Design review of the part built by this model. Coordinates are the model's own, in mm. Face numbers are marked on the shaded views. A direction names the side the tool comes from. Give positions to 0.01 mm unless a question says otherwise; leave off trailing zeros. Loops run counter-clockwise (first coordinate to the right, second up) from the corner with the lowest first, then second, coordinate; pieces in that order, holes last. Notation, with made-up numbers: M 40.25,30 L 79.25,30 A25 ccw 79.25,55 Z; hole C 19,19.5 d7. An arc over 180 degrees is marked long. Answer as CSV lines item,"result".
Autodesk Inventor part; units mm, degrees
ref_plane "YZ Plane" through (0, 0, 0) normal (1, 0, 0) x (0, 1, 0)
ref_plane "XZ Plane" through (0, 0, 0) normal (0, 1, 0) x (-1, 0, 0)
ref_plane "XY Plane" through (0, 0, 0) normal (0, 0, 1) x (1, 0, 0)
sketch "Sketch1" plane through (0, 0, 0) normal (0, 1, 0) x (-1, 0, 0)
  line L0 (0, 0) -> (56, 0)
  line L1 (56, -6.2) -> (56, -90.8)
  line L2 (56, -97) -> (0, -97)
  line L3 (0, -90.8) -> (0, -6.2)
  line L4 (0, 0) -> (-3.5, 0)
  line L5 (-4.5, -1) -> (-4.5, -4.2)
  line L6 (-3.5, -5.2) -> (-1, -5.2)
  line L7 (28, 0) -> (28, -97)
  circle A0 centre (-2.5, -2.6) radius 1.5
  arc A1 (-3.5, 0) -> (-4.5, -1) centre (-3.5, -1) ccw
  arc A2 (-4.5, -4.2) -> (-3.5, -5.2) centre (-3.5, -4.2) ccw
  arc A3 (0, -6.2) -> (-1, -5.2) centre (-1, -6.2) ccw
  line L8 (56, 0) -> (59.5, 0)
  line L9 (60.5, -1) -> (60.5, -4.2)
  line L10 (59.5, -5.2) -> (57, -5.2)
  circle A4 centre (58.5, -2.6) radius 1.5
  arc A5 (60.5, -1) -> (59.5, 0) centre (59.5, -1) ccw
  arc A6 (59.5, -5.2) -> (60.5, -4.2) centre (59.5, -4.2) ccw
  arc A7 (57, -5.2) -> (56, -6.2) centre (57, -6.2) ccw
  line L11 (56, -48.5) -> (0, -48.5)
  line L12 (0, -97) -> (-3.5, -97)
  line L13 (-4.5, -96) -> (-4.5, -92.8)
  line L14 (-3.5, -91.8) -> (-1, -91.8)
  circle A8 centre (-2.5, -94.4) radius 1.5
  arc A9 (-4.5, -96) -> (-3.5, -97) centre (-3.5, -96) ccw
  arc A10 (-3.5, -91.8) -> (-4.5, -92.8) centre (-3.5, -92.8) ccw
  arc A11 (-1, -91.8) -> (0, -90.8) centre (-1, -90.8) ccw
  arc A12 (56, -90.8) -> (57, -91.8) centre (57, -90.8) ccw
  line L15 (59.5, -91.8) -> (57, -91.8)
  line L16 (56, -97) -> (59.5, -97)
  circle A13 centre (58.5, -94.4) radius 1.5
  arc A14 (60.5, -92.8) -> (59.5, -91.8) centre (59.5, -92.8) ccw
  line L17 (60.5, -96) -> (60.5, -92.8)
  arc A15 (59.5, -97) -> (60.5, -96) centre (59.5, -96) ccw
  point P0 (-4.5, 0)
  point P1 (-4.5, -5.2)
  point P2 (0, -5.2)
  point P3 (60.5, 0)
  point P4 (60.5, -5.2)
  point P5 (56, -5.2)
  point P6 (-4.5, -97)
  point P7 (-4.5, -91.8)
  point P8 (0, -91.8)
  point P9 (56, -91.8)
  point P10 (60.5, -91.8)
  point P11 (60.5, -97)
  dimension "d0" = 56
  dimension "d1" = 97
  dimension "d2" = 4.5
  dimension "d3" = 5.2
  dimension "d10" = 1
  dimension "d11" = 1
  dimension "d12" = 2
  dimension "d13" = 2.6
  dimension "d14" = 3
  dimension "d15" = 56
extrude "Vetronite" add sketch "Sketch1" along normal blind 1.7
sketch "Sketch2" plane through (0, 1.7, 0) normal (0, 1, 0) x (1, 0, 0)
  line L0 (-59.5, 0) -> (3.5, 0)
  line L1 (-28, 0) -> (-28, 97)
  line L2 (3.5, 97) -> (-59.5, 97)
  line L3 (-56, 90.8) -> (-56, 6.2)
  line L4 (-56, 48.5) -> (0, 48.5)
  line L5 (0, 6.2) -> (0, 90.8)
  line L6 (-56, 6) -> (0, 6)
  line L7 (0, 6) -> (0, 91)
  line L8 (0, 91) -> (-56, 91)
  line L9 (-56, 91) -> (-56, 6)
  point P0 (0, 0)
  point P1 (-56, 6.2)
  dimension "d16" = 85
  dimension "d17" = 56
extrude "Display" add sketch "Sketch2" along normal blind 3.6
sketch "Sketch3" plane through (0, 0, 0) normal (0, -1, 0) x (1, 0, 0)
  line L0 (-53.3, -4) -> (-2.7, -4)
  line L1 (-2.7, -4) -> (-2.7, -1.5)
  line L2 (-2.7, -1.5) -> (-53.3, -1.5)
  line L3 (-53.3, -1.5) -> (-53.3, -4)
  line L4 (-59.5, 0) -> (3.5, 0)
  line L5 (3.5, -97) -> (-59.5, -97)
  line L6 (-28, -97) -> (-28, 0)
  line L7 (-59.5, 0) -> (3.5, 0)
  point P0 (0, 0)
  dimension "d20" = 50.6
  dimension "d21" = 2.5
  dimension "d22" = 1.5
extrude "Pin" add sketch "Sketch3" along normal blind 8.5
sketch "Sketch4" plane through (0, 0, 0) normal (0, -1, 0) x (1, 0, 0)
  line L0 (-5, -82) -> (-21, -82)
  line L1 (-21, -82) -> (-21, -68)
  line L2 (-21, -68) -> (-5, -68)
  line L3 (-5, -68) -> (-5, -82)
  line L4 (-50, -69) -> (-38, -69)
  line L5 (-38, -69) -> (-38, -57)
  line L6 (-38, -57) -> (-50, -57)
  line L7 (-50, -57) -> (-50, -69)
  line L8 (-36, -69) -> (-24, -69)
  line L9 (-24, -69) -> (-24, -57)
  line L10 (-24, -57) -> (-36, -57)
  line L11 (-36, -57) -> (-36, -69)
  line L12 (-43, -40) -> (-13, -40)
  line L13 (-13, -40) -> (-13, -24)
  line L14 (-13, -24) -> (-43, -24)
  line L15 (-43, -24) -> (-43, -40)
  line L16 (3.5, -97) -> (-59.5, -97)
  line L17 (0, -6.2) -> (0, -90.8)
  line L18 (-56, -90.8) -> (-56, -6.2)
  point P0 (0, 0)
  dimension "d25" = 16
  dimension "d26" = 14
  dimension "d27" = 12
  dimension "d28" = 12
  dimension "d29" = 12
  dimension "d30" = 12
  dimension "d31" = 30
  dimension "d32" = 16
  dimension "d33" = 15
  dimension "d34" = 5
  dimension "d35" = 28
  dimension "d36" = 6
  dimension "d37" = 2
  dimension "d38" = 57
  dimension "d40" = 13
extrude "Componenti" add sketch "Sketch4" along normal blind 2.5
draft "ScreenCables" angle 80 pull direction (0, -1, 0) faces at (-23, -0.8333, -24) fixed edges at (-28, 0, -24)
properties part number "TouchLCD" material "Lead"
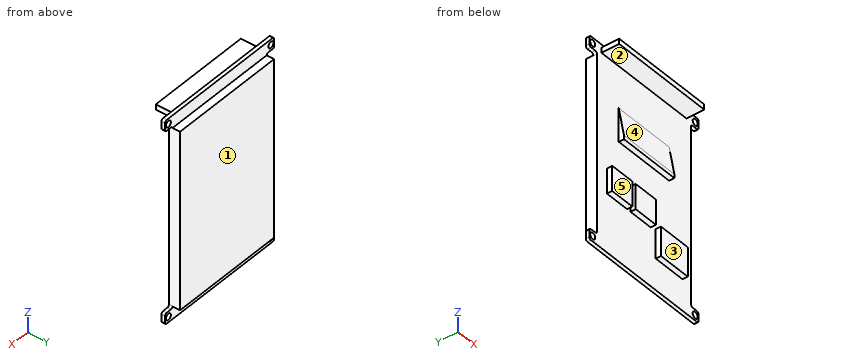
1. The part is to be moulded in two halves that separate along Z. For the marked faces 4 and 5, say which applies: pulls with the +Z half, pulls with the -Z half, needs draft (parallel to the pull), parting line crosses it, or undercut.
Answer block:
face 4,"undercut"
face 5,"needs draft"
2. For the marked faces 1, 2 and 3, list the 3-axis set-ups (+Z, -Z, +X, -X, +Y, -Y) from which the entire face can be reached by the end or side of a thin tool; tool diameter is ignored.
Answer block:
face 1,"+Z, -Z, +X, -X, +Y"
face 2,"+X, -X, -Y"
face 3,"-Z, +X, -X, -Y"
3. We need section A-A, the plane z = -94.4. Write out the cut boundary in (x, y), plus the area to 3 significant figures.
Answer block:
outline,"M -60.5,0 L -60,0 L -60,1.7 L -60.5,1.7 Z; M -57,0 L 1,0 L 1,1.7 L -57,1.7 Z; M 4,0 L 4.5,0 L 4.5,1.7 L 4,1.7 Z"
area,"100 mm²"
4. We need section B-B, the plane x = -58.5. Write out the cut boundary in (y, z), plus the area to 3 significant figures.
Answer block:
outline,"M 0,-97 L 1.7,-97 L 1.7,-95.9 L 0,-95.9 Z; M 0,-92.9 L 1.7,-92.9 L 1.7,-91.8 L 0,-91.8 Z; M 0,-5.2 L 1.7,-5.2 L 1.7,-4.1 L 0,-4.1 Z; M 0,-1.1 L 1.7,-1.1 L 1.7,0 L 0,0 Z"
area,"7.48 mm²"
5. For P1, Ø1.9, axis at x = -13.5, z = -2.5, coming from the +Y side; P2, Ø0.8, axis at y = -3.5, z = -2, coming from the -X side; P3, Ø3, axis at y = -1, z = -63.5, coming from the +X side, all flat-tipped, find the tip position at first contact; note any pin that passes through.
Answer block:
P1,"y = 1.7"
P2,"x = -53.3"
P3,"x = 0"
6. We need section D-D, the plane z = -79.5. Write out the cut boundary in (x, y).
Answer block:
outline,"M -56,0 L -21,0 L -21,-2.5 L -5,-2.5 L -5,0 L 0,0 L 0,5.3 L -56,5.3 Z"
7. We need section C-C, the plane x = -46.5. Write out the cut boundary in (y, z), plus the area to 3 significant figures.
Answer block:
outline,"M -8.5,-4 L 0,-4 L 0,-57 L -2.5,-57 L -2.5,-69 L 0,-69 L 0,-97 L 1.7,-97 L 1.7,-91 L 5.3,-91 L 5.3,-6 L 1.7,-6 L 1.7,0 L 0,0 L 0,-1.5 L -8.5,-1.5 Z"
area,"522 mm²"
8. To check wall thickness, follow L1, parallel to Z at x = 2.5, y = 0.85; L2, parallel to X at y = 1.2, z = -94.4; L3, parallel to X at y = 4, z = -53. State the ranges of each line that lie inside material, in increasing order. Write a range as [from, to].
Answer block:
L1,"[-97, -95.9], [-92.9, -91.8], [-5.2, -4.1], [-1.1, 0]"
L2,"[-60.5, -60], [-57, 1], [4, 4.5]"
L3,"[-56, 0]"
